from build123d import *

# Parameters (mm, degrees)
SKETCH1_W           = 88.9
SKETCH1_H           = 57.15
BOSS_EXTRUDE1_DEPTH = 6.35
CUT_EXTRUDE1_REACH  = 55.223
SKETCH2_R           = 8.5


with BuildPart() as part:
    # Sketch1 → Boss-Extrude1 (new body)
    with BuildSketch(Plane.XY):
        Rectangle(SKETCH1_W, SKETCH1_H)
    extrude(amount=BOSS_EXTRUDE1_DEPTH)

    # Sketch2 → Cut-Extrude1 (cut, up to next)
    with BuildSketch(Plane.XY.offset(6.35), mode=Mode.PRIVATE) as cut_extrude1_sk1:
        with Locations((0, -3.175)):
            Circle(SKETCH2_R)
    cut_extrude1_tool1 = extrude(cut_extrude1_sk1.sketch, amount=-CUT_EXTRUDE1_REACH, mode=Mode.PRIVATE) & part.part
    add(cut_extrude1_tool1.solids().sort_by_distance((0, -3.175, 6.35))[0], mode=Mode.SUBTRACT)


solid = part.part
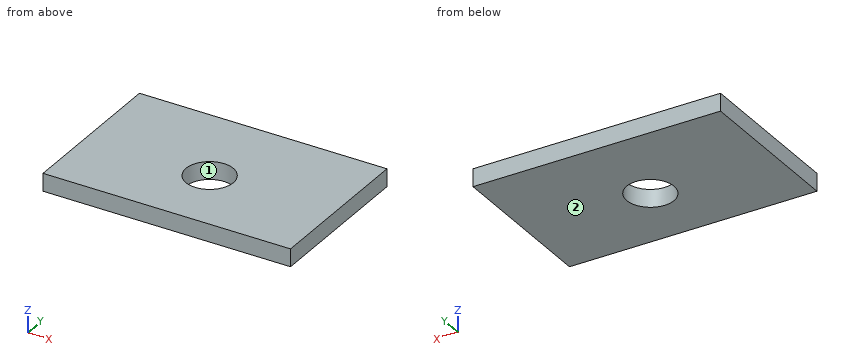
Model file for the job. Use its own axes, mm. Face numbers are marked on the shaded views. Give positions to 0.01 mm unless a question says otherwise; leave off trailing zeros. Order: outer loops, then holes, each group sorted by start corner. A loop starts at its lowest first (then second) coordinate and runs counter-clockwise, first axis right, second up. Notation, with made-up numbers: (-8, 86) - (42, 86) arc R21 ccw to (42, 99) - close; hole circle Ø2 at (2, 69.5). An arc over 180 degrees is marked (long way). Write item = value, one per line. Start each with the question number.
1. Cut at B-B, the plane y = 4. List the corners of the cut face in (x, z).
2. Two-plate mould, pull along X, no slides. Class the marked faces 1 and 2: pulls with the +X half, pulls with the -X half, needs draft (parallel to the pull), parting line crosses it, or undercut.
3. Probe line 1 along Y through (x, z) = (0, 3.25) (3 decimals); line 2 along X through (y, z) = (3.5, 5.25); line 3 along Y through (x, z) = (6, 1.5) (3 decimals). List the from-to ranges inside material, lowest first.
4. Cut at C-C, the plane z = 4. List the corners of the cut face in (x, y) (3 decimals), and give its area (3 significant figures).
5. Cut at A-A, the plane x = 0. List the corners of the cut face in (y, z) (3 decimals).
Taken from the geometry:
q1.outline = (-44.45, 0) - (-4.56, 0) - (-4.56, 6.35) - (-44.45, 6.35) - close; (4.56, 0) - (44.45, 0) - (44.45, 6.35) - (4.56, 6.35) - close
q2.face_1 = undercut
q2.face_2 = needs draft
q3.line_1 = -28.575 to -11.675, 5.325 to 28.575
q3.line_2 = -44.45 to -5.26, 5.26 to 44.45
q3.line_3 = -28.575 to -9.196, 2.846 to 28.575
q4.outline = (-44.45, -28.575) - (44.45, -28.575) - (44.45, 28.575) - (-44.45, 28.575) - close; hole circle Ø17 at (0, -3.175)
q4.area = 4,850 mm²
q5.outline = (-28.575, 0) - (-11.675, 0) - (-11.675, 6.35) - (-28.575, 6.35) - close; (5.325, 0) - (28.575, 0) - (28.575, 6.35) - (5.325, 6.35) - close
